Read the model definition and answer for the solid it produces. Units are mm, in the model's axes. A direction names the side the tool comes from. Give positions to 0.01 mm unless a question says otherwise; leave off trailing zeros. Loops run counter-clockwise (first coordinate to the right, second up) from the corner with the lowest first, then second, coordinate; pieces in that order, holes last. Notation, with made-up numbers: (-16, 32) -> (-2, 32) arc R25 cw to (-2, 67) -> close; hole circle Ø2 at (-17.75, 87). An arc over 180 degrees is marked (long way). Write each question's results on one line, items separated by ' | '. Start each with the question number.
Item 1: Find the intervals of material crossed by line 1 (X direction, y = 0.65, z = -1.5); line 2 (X direction, y = 1.2, z = 0); line 3 (X direction, y = 0.9, z = -38.4), in increasing order.
Item 2: Which of the six approach directions +Z, -Z, +X, -X, +Y, -Y give full straight-line access (tool end or side, diameter ignored) to faces 4 (the cylindrical face through (37.14, 1.48, -10.5)), 5 (the cylindrical face through (-10.73, 2.57, 10.43))?
Item 3: Section A-A on x = 30 is taken. Write down the section's boundary in (y, z).
Item 4: Determine the mould class of faces 1 (the cylindrical face through (-41.688, 1.479, -27.617)), 2 (the cylindrical face through (27.617, 1.479, -41.688)), 3 (the cylindrical face through (-17.61, 1.48, 17.3)) for opening direction X: +X half, -X half, draft (parallel to the pull), parting line (faces both ways), or undercut.
Item 5: Section B-B on z = -2 is taken. Write down the section's boundary in (x, y), and give its area (3 significant figures).
Item 6: Each of these flat-tipped pins is pushed along its axis until it touches: P1, Ø1.5, axis at x = -18, z = -23, coming from the -Y side; P2, Ø0.8, axis at x = -34.5, y = 2, coming from the +Z side; P3, Ø0.9, axis at y = 2, z = -31, coming from the -X side; P4, Ø1.5, axis at x = 28.5, y = 2, coming from the +Z side. Where does it stop, or does it pass through?
```python
from build123d import *

# Parameters (mm, degrees)
SKETCH1_W           = 86
SKETCH1_H           = 86
BOSS_EXTRUDE1_DEPTH = 3
SKETCH2_R           = 8.5
SKETCH2_W           = 14
SKETCH2_H           = 14
CUT_EXTRUDE1_DEPTH  = 61.88513776
FILLET1_R           = 4.6
FILLET2_R           = 5
SKETCH3_R           = 2.1
CUT_EXTRUDE2_DEPTH  = 61.88513776
SKETCH4_W           = 23.5
SKETCH4_H           = 22.8
SKETCH4_R           = 8.5
CUT_EXTRUDE3_DEPTH  = 0.85
FILLET3_R           = 3.4
SKETCH5_W           = 23.5
SKETCH5_H           = 14
SKETCH5_H_2         = 7.6
SKETCH5_W_2         = 14
SKETCH5_H_3         = 22.8
SKETCH5_W_3         = 7.25
CUT_EXTRUDE4_DEPTH  = 61.88513776
FILLET4_R           = 3


with BuildPart() as part:
    # Sketch1 → Boss-Extrude1 (new body)
    with BuildSketch(Plane(origin=(0, 0, 0), x_dir=(1, 0, 0), z_dir=(0, 1, 0))):
        Rectangle(SKETCH1_W, SKETCH1_H)
    extrude(amount=BOSS_EXTRUDE1_DEPTH)

    # Sketch2 → Cut-Extrude1 (cut, through all)
    with BuildSketch(Plane(origin=(0, 3, 0), x_dir=(1, 0, 0), z_dir=(0, 1, 0))):
        with Locations(Location((0, 0, 0), (0, 0, 270))):
            Circle(SKETCH2_R)
        with Locations((36, 36)):
            Rectangle(SKETCH2_W, SKETCH2_H)
        with Locations((-36, 36)):
            Rectangle(SKETCH2_W, SKETCH2_H)
        with Locations((36, -36)):
            Rectangle(SKETCH2_W, SKETCH2_H)
        with Locations((-36, -36)):
            Rectangle(SKETCH2_W, SKETCH2_H)
    extrude(amount=-CUT_EXTRUDE1_DEPTH, mode=Mode.SUBTRACT)

    # Fillet1
    fillet1_edges = [part.edges().sort_by_distance(p)[0] for p in [
        (-43, 1.5, 29),
        (-29, 1.5, 43),
        (43, 1.5, 29),
        (29, 1.5, 43),
        (29, 1.5, -43),
        (43, 1.5, -29),
        (-43, 1.5, -29),
        (-29, 1.5, -43),
    ]]
    fillet(fillet1_edges, radius=FILLET1_R)

    # Fillet2
    fillet2_edges = [part.edges().sort_by_distance(p)[0] for p in [
        (-29, 1.5, 29),
        (29, 1.5, 29),
        (29, 1.5, -29),
        (-29, 1.5, -29),
    ]]
    fillet(fillet2_edges, radius=FILLET2_R)

    # Sketch3 → Cut-Extrude2 (cut, through all)
    with BuildSketch(Plane(origin=(0, 3, 0), x_dir=(1, 0, 0), z_dir=(0, 1, 0))):
        with Locations(Location((38.4, 24.4, 0), (0, 0, 270))):
            Circle(SKETCH3_R)
        with Locations(Location((-24.4, 38.4, 0), (0, 0, 270))):
            Circle(SKETCH3_R)
        with Locations(Location((24.4, -38.4, 0), (0, 0, 270))):
            Circle(SKETCH3_R)
        with Locations(Location((-38.4, -24.4, 0), (0, 0, 270))):
            Circle(SKETCH3_R)
    extrude(amount=-CUT_EXTRUDE2_DEPTH, mode=Mode.SUBTRACT)

    # Sketch4 → Cut-Extrude3 (cut)
    with BuildSketch(Plane(origin=(0, 3, 0), x_dir=(1, 0, 0), z_dir=(0, 1, 0))):
        Rectangle(SKETCH4_W, SKETCH4_H)
        with Locations(Location((0, 0, 0), (0, 0, 270))):
            Circle(SKETCH4_R, mode=Mode.SUBTRACT)
    extrude(amount=-CUT_EXTRUDE3_DEPTH, mode=Mode.SUBTRACT)

    # Fillet3
    fillet3_edges = [part.edges().sort_by_distance(p)[0] for p in [
        (-11.75, 2.575, 11.4),
        (-11.75, 2.575, -11.4),
        (11.75, 2.575, -11.4),
        (11.75, 2.575, 11.4),
    ]]
    fillet(fillet3_edges, radius=FILLET3_R)

    # Sketch5 → Cut-Extrude4 (cut, through all)
    with BuildSketch(Plane(origin=(0, 3, 0), x_dir=(1, 0, 0), z_dir=(0, 1, 0))):
        with Locations((0, 31)):
            Rectangle(SKETCH5_W, SKETCH5_H)
        with Locations((0, 20.2)):
            Rectangle(SKETCH5_W, SKETCH5_H_2)
        with Locations((-31, 0)):
            Rectangle(SKETCH5_W_2, SKETCH5_H_3)
        with Locations((-20.375, 0)):
            Rectangle(SKETCH5_W_3, SKETCH5_H_3)
        with Locations((31, 0)):
            Rectangle(SKETCH5_W_2, SKETCH5_H_3)
        with Locations((20.375, 0)):
            Rectangle(SKETCH5_W_3, SKETCH5_H_3)
        with Locations((0, -20.2)):
            Rectangle(SKETCH5_W, SKETCH5_H_2)
        with Locations((0, -31)):
            Rectangle(SKETCH5_W, SKETCH5_H)
        with Locations((20.375, -20.2)):
            Rectangle(SKETCH5_W_3, SKETCH5_H_2)
        Polygon((24, -16.4), (24, -24), (34, -24), (38, -24), (38, -16.4), align=None)
        with BuildLine():
            Line((24, -24), (16.75, -24))
            Line((16.75, -24), (16.75, -38))
            Line((16.75, -38), (17.311276561, -38))
            ThreePointArc((17.311276561, -38), (19.379541854, -33.379541854), (24, -31.311276561))
            Line((24, -31.311276561), (24, -24))
        make_face()
        with BuildLine():
            Line((34, -24), (24, -24))
            Line((24, -24), (24, -31.311276561))
            ThreePointArc((24, -31.311276561), (24.185616902, -31.303237366), (24.371380604, -31.300057681))
            ThreePointArc((24.371380604, -31.300057681), (27.958453145, -26.031329371), (34, -24))
        make_face()
        Polygon((-16.75, -24), (-24, -24), (-24, -34), (-24, -38), (-16.75, -38), align=None)
        with Locations((-20.375, -20.2)):
            Rectangle(SKETCH5_W_3, SKETCH5_H_2)
        with BuildLine():
            Line((-24, -24), (-24, -16.4))
            Line((-24, -16.4), (-38, -16.4))
            Line((-38, -16.4), (-38, -17.311276561))
            ThreePointArc((-38, -17.311276561), (-33.379541854, -19.379541854), (-31.311276561, -24))
            Line((-31.311276561, -24), (-24, -24))
        make_face()
        with BuildLine():
            Line((-24, -34), (-24, -24))
            Line((-24, -24), (-31.311276561, -24))
            ThreePointArc((-31.311276561, -24), (-31.303237366, -24.185616902), (-31.300057681, -24.371380604))
            ThreePointArc((-31.300057681, -24.371380604), (-26.031329371, -27.958453145), (-24, -34))
        make_face()
        Polygon((-38, 16.4), (-24, 16.4), (-24, 24), (-34, 24), (-38, 24), align=None)
        with BuildLine():
            Line((-24, 31.311276561), (-24, 24))
            Line((-24, 24), (-16.75, 24))
            Line((-16.75, 24), (-16.75, 38))
            Line((-16.75, 38), (-17.311276561, 38))
            ThreePointArc((-17.311276561, 38), (-19.379541854, 33.379541854), (-24, 31.311276561))
        make_face()
        with Locations((-20.375, 20.2)):
            Rectangle(SKETCH5_W_3, SKETCH5_H_2)
        with BuildLine():
            Line((-34, 24), (-24, 24))
            Line((-24, 24), (-24, 31.311276561))
            ThreePointArc((-24, 31.311276561), (-24.185616902, 31.303237366), (-24.371380604, 31.300057681))
            ThreePointArc((-24.371380604, 31.300057681), (-27.958453145, 26.031329371), (-34, 24))
        make_face()
        Polygon((16.75, 38), (16.75, 24), (24, 24), (24, 34), (24, 38), align=None)
        with Locations((20.375, 20.2)):
            Rectangle(SKETCH5_W_3, SKETCH5_H_2)
        with BuildLine():
            Line((31.311276561, 24), (24, 24))
            Line((24, 24), (24, 16.4))
            Line((24, 16.4), (38, 16.4))
            Line((38, 16.4), (38, 17.311276561))
            ThreePointArc((38, 17.311276561), (33.379541854, 19.379541854), (31.311276561, 24))
        make_face()
        with BuildLine():
            Line((24, 34), (24, 24))
            Line((24, 24), (31.311276561, 24))
            ThreePointArc((31.311276561, 24), (31.303237366, 24.185616902), (31.300057681, 24.371380604))
            ThreePointArc((31.300057681, 24.371380604), (26.031329371, 27.958453145), (24, 34))
        make_face()
    extrude(amount=-CUT_EXTRUDE4_DEPTH, mode=Mode.SUBTRACT)

    # Fillet4
    fillet4_edges = [part.edges().sort_by_distance(p)[0] for p in [
        (-16.75, 1.5, 11.4),
        (-38, 1.5, 11.4),
        (-38, 1.5, -11.4),
        (-16.75, 1.5, -11.4),
        (16.75, 1.5, -11.4),
        (38, 1.5, -11.4),
        (38, 1.5, 11.4),
        (16.75, 1.5, 11.4),
        (-11.75, 1.5, 38),
        (-11.75, 1.5, 16.4),
        (11.75, 1.5, 16.4),
        (11.75, 1.5, 38),
        (16.75, 1.5, 16.4),
        (38, 1.5, 16.4),
        (-16.75, 1.5, 16.4),
        (-16.75, 1.5, 38),
        (-24, 1.5, 38),
        (-38, 1.5, -24),
        (-16.75, 1.5, -16.4),
        (-38, 1.5, -16.4),
        (16.75, 1.5, -16.4),
        (16.75, 1.5, -38),
        (24, 1.5, -38),
        (-11.75, 1.5, -16.4),
        (-11.75, 1.5, -38),
        (11.75, 1.5, -38),
        (11.75, 1.5, -16.4),
    ]]
    fillet(fillet4_edges, radius=FILLET4_R)


solid = part.part
```
Findings:
1) line 1: -43 to -38, -16.75 to -8.37, 8.37 to 16.75, 38 to 43 | line 2: -43 to -38, -16.75 to -8.5, 8.5 to 16.75, 38 to 43 | line 3: -29 to -26.5, -22.3 to 29
2) face 4: +Y, -Y | face 5: +Y
3) outline: (0, -31) -> (3, -31) -> (3, -24.83) -> (0, -24.83) -> close; (0, -16.4) -> (3, -16.4) -> (3, -11.4) -> (0, -11.4) -> close; (0, 11.4) -> (3, 11.4) -> (3, 16.4) -> (0, 16.4) -> close; (0, 24.83) -> (3, 24.83) -> (3, 31) -> (0, 31) -> close
4) face 1: -X half | face 2: +X half | face 3: undercut
5) outline: (-43, 0) -> (-38, 0) -> (-38, 3) -> (-43, 3) -> close; (-16.75, 0) -> (-8.26, 0) -> (-8.26, 2.15) -> (-11.75, 2.15) -> (-11.75, 3) -> (-16.75, 3) -> close; (8.26, 0) -> (16.75, 0) -> (16.75, 3) -> (11.75, 3) -> (11.75, 2.15) -> (8.26, 2.15) -> close; (38, 0) -> (43, 0) -> (43, 3) -> (38, 3) -> close | area: 75.0 mm2
6) P1: through | P2: z = 29 | P3: x = -30.38 | P4: z = 41.55
